```python
from build123d import *

# Parameters (mm, degrees)
SKETCH_1_R          = 1
EXTRUDE_1_DEPTH     = 2.1
CUT_EXTRUDE_2_DEPTH = 1.5
EXTRUDE_START       = 5
SKETCH_4_R          = 8
EXTRUDE_2_DEPTH     = 5
CUT_EXTRUDE_3_DEPTH = 63.152312909
SKETCH_2_R          = 1.1
CUT_EXTRUDE_1_DEPTH = 63.152312909
SKETCH_6_R          = 2.5
CUT_EXTRUDE_4_DEPTH = 5


with BuildPart() as part:
    # 草图1 → 凸台-拉伸1 (new body)
    with BuildSketch(Plane(origin=(0, 0, 0), x_dir=(1, 0, 0), z_dir=(0, 1, 0))):
        with BuildLine():
            Line((-25.678571429, 20.478304847), (3.314285714, 7.281175057))
            ThreePointArc((3.314285714, 7.281175057), (8, 0), (3.314285714, -7.281175057))
            Line((3.314285714, -7.281175057), (-25.678571429, -20.478304847))
            ThreePointArc((-25.678571429, -20.478304847), (-57.5, 0), (-25.678571429, 20.478304847))
        make_face()
        with Locations(Location((0, 0, 0), (0, 0, 270))):
            Circle(SKETCH_1_R, mode=Mode.SUBTRACT)
    extrude(amount=EXTRUDE_1_DEPTH)

    # 草图3 → 切除-拉伸2 (cut)
    with BuildSketch(Plane(origin=(0, 2.1, 0), x_dir=(1, 0, 0), z_dir=(0, 1, 0))):
        with BuildLine():
            Line((-5.361902647, 4.5), (0, 4.5))
            ThreePointArc((0, 4.5), (4.5, 0), (0, -4.5))
            Line((0, -4.5), (-5.361902647, -4.5))
            ThreePointArc((-5.361902647, -4.5), (-7, 0), (-5.361902647, 4.5))
        make_face()
    extrude(amount=-CUT_EXTRUDE_2_DEPTH, mode=Mode.SUBTRACT)

    # 草图4 → 凸台-拉伸2 (add)
    with BuildSketch(Plane.XZ.offset(EXTRUDE_START)):
        with Locations(Location((0, 0, 0), (0, 0, 270))):
            Circle(SKETCH_4_R)
    extrude(amount=-EXTRUDE_2_DEPTH)

    # 草图5 → 切除-拉伸3 (cut, through all)
    with BuildSketch(Plane.XZ.offset(5)):
        Polygon((1, -1), (1, -3.5), (-1, -3.5), (-1, -1), (-3.5, -1), (-3.5, 1), (-1, 1), (-1, 3.5), (1, 3.5), (1, 1), (3.5, 1), (3.5, -1), align=None)
    extrude(amount=-CUT_EXTRUDE_3_DEPTH, mode=Mode.SUBTRACT)

    # 草图2 → 切除-拉伸1 (cut, through all)
    with BuildSketch(Plane(origin=(0, 2.1, 0), x_dir=(1, 0, 0), z_dir=(0, 1, 0))):
        with Locations(Location((-8.5, 0, 0), (0, 0, 270))):
            Circle(SKETCH_2_R)
        with Locations(Location((-16, 0, 0), (0, 0, 270))):
            Circle(SKETCH_2_R)
    extrude(amount=-CUT_EXTRUDE_1_DEPTH, mode=Mode.SUBTRACT)

    # 草图6 → 切除-拉伸4 (cut)
    with BuildSketch(Plane.XZ.offset(5)):
        with Locations((-8.5, 0)):
            Circle(SKETCH_6_R)
    extrude(amount=-CUT_EXTRUDE_4_DEPTH, mode=Mode.SUBTRACT)


solid = part.part
```
Build history of the part. All positions in model axes, mm. A direction names the side the tool comes from. Coordinates: 2 decimals unless noted, no trailing zeros. Order: outer loops, then holes, each group sorted by start corner. A loop starts at its lowest first (then second) coordinate and runs counter-clockwise, first axis right, second up. Notation, with made-up numbers: M 4,76 L 52,76 A29 cw 52,111 Z; hole C 49.5,-5 d5. An arc over 180 degrees is marked long. One line per question, with ' | ' between items. Start each with the question number.
1. Cut at D-D (x = -23). Write the cut outline in (y, z), plus the area to 3 significant figures.
2. Mould opens along X. For faces 4 (the face through (2, -2, 1)), 5 (the face through (-57.49, 1.04, 0.63)), 6 (the face through (-33, 0, 0)), 7 (the face through (-3, 1, 4.5)) say: +X half, -X half, draft (parallel to the pull), parting line (faces both ways), or undercut.
3. Cut at B-B (x = -2.5). Write the cut outline in (y, z), plus the area to 3 significant figures.
4. Tool access for faces 1 (the face through (4.5, 1.4, -0.1)), 2 (the face through (-11.385, 1.035, -13.972)), 3 (the face through (-3.5, -2, 0)): list every direction of +Z, -Z, +X, -X, +Y, -Y with a clear straight run to the whole face (end or side of a thin tool).
5. Cut at A-A (z = 0). Write the cut outline in (x, y), plus the area to 3 significant figures.
6. Cut at C-C (y = -2.75). Write the cut outline in (x, z).
7. Flat gauge pins, fed straight in: P1, Ø0.6, axis at y = -1, z = 0.5, coming from the +X side; P2, Ø22.5, axis at x = -40, z = -10.5, coming from the -Y side; P3, Ø1.2, axis at y = -3, z = -2.5, coming from the +X side. Where does each tip first touch, or does it go through?
8. Wall check: line 1 along Y through (x, z) = (-11, -10.5); line 2 along Z through (x, y) = (2, -2.25); line 3 along Z through (x, y) = (-10, 1.5). Give the ranges that are in metal, low to high. Write a range as [from, to].
The answers:
1) outline: M 0,-19.26 L 2.1,-19.26 L 2.1,19.26 L 0,19.26 Z | area: 80.9 mm2
2) face 4: undercut | face 5: parting line | face 6: draft | face 7: undercut
3) outline: M -5,-7.6 L 0,-7.6 L 0,-9.93 L 2.1,-9.93 L 2.1,-4.5 L 0.6,-4.5 L 0.6,-1 L -5,-1 Z; M -5,1 L 0.6,1 L 0.6,4.5 L 2.1,4.5 L 2.1,9.93 L 0,9.93 L 0,7.6 L -5,7.6 Z | area: 93.0 mm2
4) face 1: +Y | face 2: -Z, +X, +Y, -Y | face 3: +Y, -Y
5) outline: M -57.5,0 L -17.1,0 L -17.1,2.1 L -57.5,2.1 Z; M -14.9,0 L -9.6,0 L -9.6,2.1 L -14.9,2.1 Z; M -7.4,0 L -6,0 L -6,-5 L -3.5,-5 L -3.5,0.6 L -7,0.6 L -7,2.1 L -7.4,2.1 Z; M 3.5,-5 L 8,-5 L 8,2.1 L 4.5,2.1 L 4.5,0.6 L 3.5,0.6 Z | area: 142 mm2
6) outline: M -7.65,-2.35 A8 ccw long -7.65,2.35 A2.5 cw Z; hole M -3.5,-1 L -1,-1 L -1,-3.5 L 1,-3.5 L 1,-1 L 3.5,-1 L 3.5,1 L 1,1 L 1,3.5 L -1,3.5 L -1,1 L -3.5,1 Z
7) P1: stops at x = 8 | P2: stops at y = 0 | P3: stops at x = 7.77
8) line 1: y = [0, 2.1] | line 2: z = [-7.75, -1], [1, 7.75] | line 3: z = [-13.34, 13.34]
